from build123d import *

# Parameters (mm, degrees)
REDONDEO1_R                      = 0.762
TALADRO_DE_MARGEN_PARA_101_D     = 1.4986
TALADRO_DE_MARGEN_PARA_101_DEPTH = 1.1176
TALADRO_DE_MARGEN_PARA_101_TIP   = 0.450224862
CHAFL_N1_SIZE                    = 0.8382
CHAFL_N1_SIZE2                   = 0.483934996


with BuildPart() as part:
    # Croquis1 → Revolución1 (revolve)
    with BuildSketch(Plane(origin=(0, 0, 0), x_dir=(0, 0, -1), z_dir=(1, 0, 0)), mode=Mode.PRIVATE) as revoluci_n1_sk:
        Polygon((-13.4874, 0), (-13.4874, 1.9812), (0.1524, 1.9812), (0.1524, 1.8542), (0.2794, 1.8542), (0.2794, 1.9812), (3.3274, 1.9812), (3.3274, 1.7653), (13.4874, 1.7653), (13.4874, 0), align=None)
    revolve(revoluci_n1_sk.sketch.rotate(Axis((0, 0, 127), (0, 0, -1)), 90), axis=Axis((0, 0, 127), (0, 0, -1)))

    # Redondeo1
    # the kernel refuses this fillet: 0.762 mm, written as the material it adds along each edge
    with BuildSketch(Plane(origin=(0, 0, -3.3274), x_dir=(1, 0, 0), z_dir=(0, 1, 0))) as redondeo1_piece_1:
        with BuildLine():
            CenterArc((2.5273, 0.531430889), REDONDEO1_R, 180, 44.220044428)
            Line((1.7653, 0.531430889), (1.75006, 0.531430889))
            Line((1.75006, 0.531430889), (1.75006, 0))
            Line((1.75006, 0), (1.7653, -0.01524))
            ThreePointArc((1.7653, -0.01524), (1.87325, -0.01524), (1.970278, -0.010628618))
            Line((1.970278, -0.010628618), (1.9812, 0))
        make_face()
    revolve(axis=Axis((0, 0, -3.3274), (0, 0, -1)))

    # Taladro de margen para #101
    with Locations(Plane(origin=(0, 0, -13.4874), x_dir=(-1, 0, 0), z_dir=(0, 0, -1))):
        with Locations((0, 0)):
            Hole(TALADRO_DE_MARGEN_PARA_101_D / 2, depth=TALADRO_DE_MARGEN_PARA_101_DEPTH)
            with Locations((0, 0, -(TALADRO_DE_MARGEN_PARA_101_DEPTH + TALADRO_DE_MARGEN_PARA_101_TIP / 2))):  # 118° drill point
                Cone(0, TALADRO_DE_MARGEN_PARA_101_D / 2, TALADRO_DE_MARGEN_PARA_101_TIP, mode=Mode.SUBTRACT)

    # Chaflán1
    chafl_n1_edges = [part.edges().sort_by_distance(p)[0] for p in [
        (-0.7493, 0, -13.4874),
    ]]
    chafl_n1_side = [part.faces().sort_by_distance(p)[0] for p in [
        (-1.715369776, 0, -13.4874),
    ]]
    chamfer(chafl_n1_edges, length=CHAFL_N1_SIZE, length2=CHAFL_N1_SIZE2, reference=chafl_n1_side[0])


solid = part.part
Could you check a few things on this model? Use its own coordinates, in mm. A direction names the side the tool comes from. Coordinates: 2 decimals unless noted, no trailing zeros. Order: outer loops, then holes, each group sorted by start corner. A loop starts at its lowest first (then second) coordinate and runs counter-clockwise, first axis right, second up. Notation, with made-up numbers: (72, -29) -> (81, -29) arc R20 cw to (81, -22) -> close; hole circle Ø7 at (12.5, -40). An arc over 180 degrees is marked (long way). One line per question, with ' | ' between items.
Q1. If I drill on L1, parallel to X at y = 0, z = -12.6; L2, parallel to X at y = 0.15, z = -6, over which ranges is the centre line in solid material (lowest first)?
Return value:
L1: -1.77 to -0.75, 0.75 to 1.77 | L2: -1.76 to 1.76
Q2. Imagine slicing it at A-A on z = -8.75. Please give me the cut outline in (x, y).
Return value:
outline: circle Ø3.53 at (0, 0)
Q3. I'm going to push flat-ended pins straight in: P1, Ø2, axis at x = -1.5, z = 7, coming from the -Y side; P2, Ø0.9, axis at x = 0, y = 0, coming from the -Z side. Where does each tip first touch, or does it pass through?
Return value:
P1: y = -1.92 | P2: z = -12.19
Q4. On a 3-axis mill with a long thin cutter (end or side, diameter ignored), from which of +Z, -Z, +X, -X, +Y, -Y can I reach the whole of each face in a straight line? I mean faces 1 (the face through (0, 0, 13.487)), 2 (the face through (0.715, 0.225, -12.682)). Say none if no direction works.
Return value:
face 1: +Z, +X, -X, +Y, -Y | face 2: -Z
